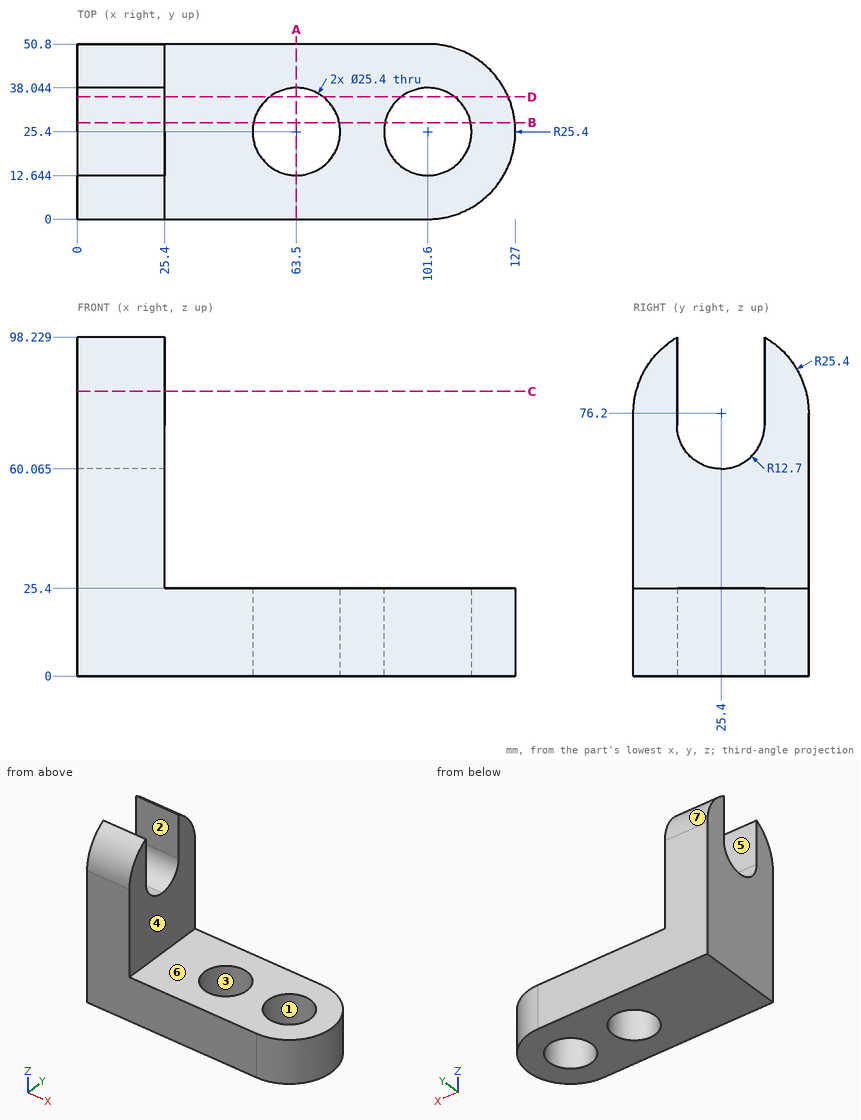
Study the drawing (mm; zero at the part's minimum x, y, z) and answer. A direction names the side the tool comes from. Round coordinates to 2 decimals unless told otherwise and drop trailing zeros. Write each loop counter-clockwise with the first axis right and the second up, starting at its lowest first coordinate (ties: lowest second). Pieces come first, ordered by that corner, then holes. Notation, with made-up numbers: (51.5, -7.5) -> (98.5, -7.5) arc R27 ccw to (98.5, 15.5) -> close; hole circle Ø9 at (37.25, 63). An arc over 180 degrees is marked (long way). Write each question's results on one line, items separated by ' | '.
Item 1: Which of the six approach directions +Z, -Z, +X, -X, +Y, -Y give full straight-line access (tool end or side, diameter ignored) to the marked faces 5, 6 and 7?
Result set:
face 5: +Z, +X, -X | face 6: +Z, +X, +Y, -Y | face 7: +Z, +X, -X, +Y
Item 2: A cutting plane is placed at D-D, the plane y = 35.5. Determine the outline of the cut face in (x, z) (1 decimal), plus the area to 3 significant figures.
Result set:
outline: (0, 0) -> (55.8, 0) -> (55.8, 25.4) -> (25.4, 25.4) -> (25.4, 65.1) -> (0, 65.1) -> close; (71.2, 0) -> (93.9, 0) -> (93.9, 25.4) -> (71.2, 25.4) -> close; (109.3, 0) -> (124.9, 0) -> (124.9, 25.4) -> (109.3, 25.4) -> close | area: 3,400 mm^2
Item 3: Find the intervals of material crossed by line 1 along X through (y, z) = (25, 14); line 2 along Y through (x, z) = (101.6, 6.75); line 3 along X through (y, z) = (27.5, 11.5) (1 decimal), in increasing order. Write a range as [from, to].
Result set:
line 1: [0, 50.81], [76.19, 88.91], [114.29, 127] | line 2: [0, 12.7], [38.1, 50.8] | line 3: [0, 51], [76, 89.1], [114.1, 126.9]
Item 4: A cutting plane is placed at B-B, the plane y = 28. Determine the outline of the cut face in (x, z) (1 decimal), plus the area to 3 significant figures.
Result set:
outline: (0, 0) -> (51.1, 0) -> (51.1, 25.4) -> (25.4, 25.4) -> (25.4, 60.3) -> (0, 60.3) -> close; (75.9, 0) -> (89.2, 0) -> (89.2, 25.4) -> (75.9, 25.4) -> close; (114, 0) -> (126.9, 0) -> (126.9, 25.4) -> (114, 25.4) -> close | area: 2,850 mm^2
Item 5: The mould has two halves that part along X. Classify the marked faces 1, 2, 3 and 4: +X half, -X half, draft (parallel to the pull), parting line (faces both ways), or undercut.
Result set:
face 1: undercut | face 2: draft | face 3: undercut | face 4: +X half
Item 6: A cutting plane is placed at A-A, the plane x = 63.5. Determine the outline of the cut face in (y, z).
Result set:
outline: (0, 0) -> (12.7, 0) -> (12.7, 25.4) -> (0, 25.4) -> close; (38.1, 0) -> (50.8, 0) -> (50.8, 25.4) -> (38.1, 25.4) -> close
Item 7: A cutting plane is placed at C-C, the plane z = 82.5. Determine the outline of the cut face in (x, y), plus the area to 3 significant figures.
Result set:
outline: (0, 0.79) -> (25.4, 0.79) -> (25.4, 12.64) -> (0, 12.64) -> close; (0, 38.04) -> (25.4, 38.04) -> (25.4, 50.01) -> (0, 50.01) -> close | area: 605 mm^2
Item 8: Flat-ended cylindrical pins translate along their axes: P1, Ø12.5, axis at x = 9.5, z = 87.5, coming from the +Y side; P2, Ø6, axis at y = 9.5, z = 17.5, coming from the +X side; P3, Ø20.5, axis at x = 63.5, y = 25.4, coming from the -Z side; P4, Ø20.5, axis at x = 16, z = 90.5, coming from the -Y side (3 decimals). Find the tip coordinate at first contact, or state that the pin passes through.
Result set:
P1: y = 50.29 | P2: x = 123.48 | P3: through | P4: y = 0.325
